Source: three-view drawing plus pictorial views. Frame: mm from the lowest corner of the part. A direction names the side the tool comes from. Round coordinates to 2 decimals unless told otherwise and drop trailing zeros. Write each loop counter-clockwise with the first axis right and the second up, starting at its lowest first coordinate (ties: lowest second). Pieces come first, ordered by that corner, then holes. Notation, with made-up numbers: M 33.25,-16 L 73.25,-16 A16 cw 73.25,12 Z; hole C 87,13.25 d7. An arc over 180 degrees is marked long. Put each result on its own line as item: value. Start each with the question number.
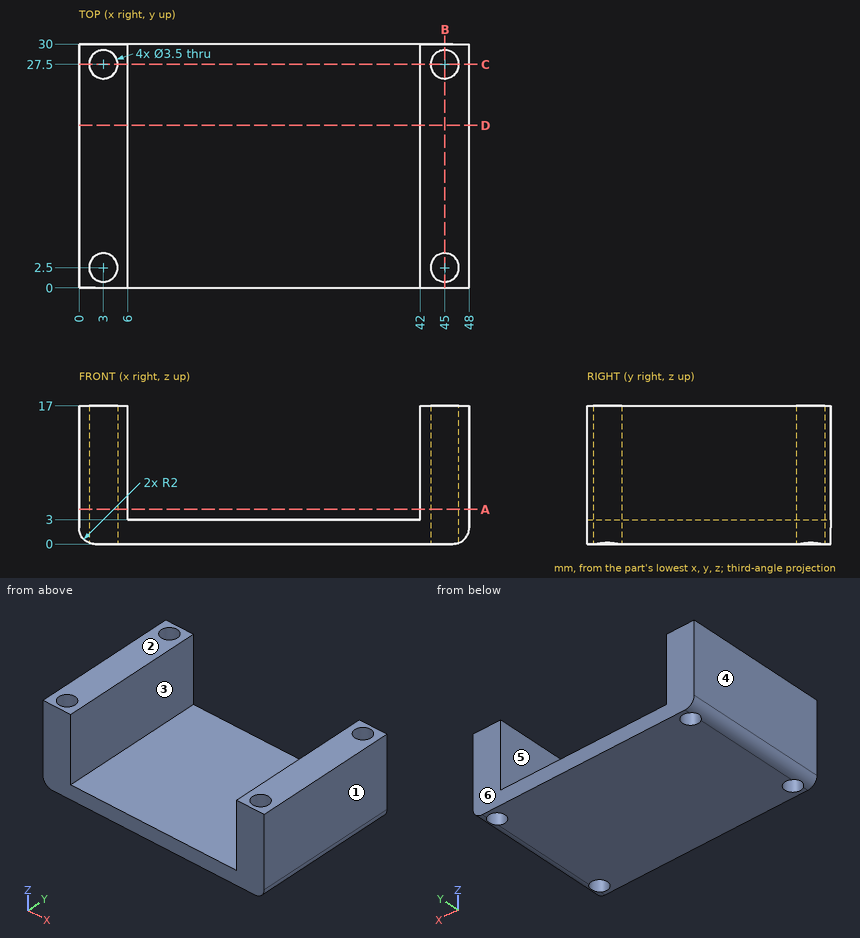
(1) Section query A-A (z = 4.25). Return loops of the section in (x, y).
(2) Section query C-C (y = 27.5). Return loops of the section in (x, z).
(3) Section query B-B (x = 45). Return loops of the section in (y, z).
(4) Section query D-D (y = 20). Return loops of the section in (x, z), and give its area (3 significant figures).
(5) Pull-direction query (X, two-part tool) for the marked faces 1, 2, 3 and 4; classes: +X half, -X half, draft (parallel to the pull), parting line (faces both ways), or undercut.
(6) Access query for the marked faces 5 and 6. Directions: +Z, -Z, +X, -X, +Y, -Y. A direction counts if a zero-diameter tool reaches every point of the face in a straight line with its end or side. Return the directions, or none.
(7) Ray query, line 1 along Y through (x, z) = (3, 11); line 2 along X through (y, z) = (6.5, 4.5); line 3 along X through (y, z) = (2, 2.75). Return the intervals inside material, ascending.
(8) Contact query for flat-ended pins moving along their axis: P1, Ø3, axis at x = 3, y = 2.5, coming from the +Z side; P2, Ø9, axis at x = 21, y = 13.5, coming from the +Z side. Output: stop coordinate, or through.
Entries:
1. outline: M 0,0 L 6,0 L 6,30 L 0,30 Z; M 42,0 L 48,0 L 48,30 L 42,30 Z; hole C 3,2.5 d3.5; hole C 3,27.5 d3.5; hole C 45,2.5 d3.5; hole C 45,27.5 d3.5
2. outline: M 0,2 A2 ccw 1.25,0.15 L 1.25,17 L 0,17 Z; M 4.75,0 L 43.25,0 L 43.25,17 L 42,17 L 42,3 L 6,3 L 6,17 L 4.75,17 Z; M 46.75,0.15 A2 ccw 48,2 L 48,17 L 46.75,17 Z
3. outline: M 0,0 L 0.75,0 L 0.75,17 L 0,17 Z; M 4.25,0 L 25.75,0 L 25.75,17 L 4.25,17 Z; M 29.25,0 L 30,0 L 30,17 L 29.25,17 Z
4. outline: M 0,2 A2 ccw 2,0 L 46,0 A2 ccw 48,2 L 48,17 L 42,17 L 42,3 L 6,3 L 6,17 L 0,17 Z
4. area: 310 mm2
5. face 1: +X half
5. face 2: draft
5. face 3: undercut
5. face 4: -X half
6. face 5: +Z, +Y, -Y
6. face 6: +Z, -Z, +X, -X, +Y
7. line 1: 0 to 0.75, 4.25 to 25.75, 29.25 to 30
7. line 2: 0 to 6, 42 to 48
7. line 3: 0 to 1.32, 4.68 to 43.32, 46.68 to 48
8. P1: through
8. P2: z = 3
